Autodesk Inventor part; units mm, degrees
ref_plane "YZ Plane" through (0, 0, 0) normal (1, 0, 0) x (0, 1, 0)
ref_plane "XZ Plane" through (0, 0, 0) normal (0, 1, 0) x (-1, 0, 0)
ref_plane "XY Plane" through (0, 0, 0) normal (0, 0, 1) x (1, 0, 0)
sketch "Sketch1" plane through (0, 0, 0) normal (1, 0, 0) x (0, 1, 0)
  circle A0 centre (0, 0) radius 2.5
  line L0 (2.3039, 4.0032) -> (4.6188, 0.0063)
  line L1 (4.6188, 0.0063) -> (2.3149, -3.9968)
  line L2 (2.3149, -3.9968) -> (-2.3039, -4.0032)
  line L3 (-2.3039, -4.0032) -> (-4.6188, -0.0063)
  line L4 (-4.6188, -0.0063) -> (-2.3149, 3.9968)
  line L5 (-2.3149, 3.9968) -> (2.3039, 4.0032)
  dimension "d0" = 5
  dimension "d1" = 8
extrude "Extrusion1" add sketch "Sketch1" along normal blind 30 contours A0
extrude "Extrusion2" add sketch "Sketch1" against normal blind 5 contours A0 | L0 L1 L2 L3 L4 L5
thread "Thread1"
fillet "Fillet1" radius 0.5 6 edges at (-2.5, 2.3039, 4.0032) (-2.5, 4.6188, 0.0063) (-2.5, -2.3149, 3.9968) (-2.5, -4.6188, -0.0063) (-2.5, -2.3039, -4.0032) (-2.5, 2.3149, -3.9968)
fillet "Fillet2" radius 0.5 24 edges at (-5, -4.5414, -0.0062) (-5, -3.4668, 1.9953) (-5, -2.2761, 3.9299) (-5, -0.0055, 4) (-5, 2.2653, 3.9361) (-5, 3.4614, 2.0047) (-5, 4.5414, 0.0062) (-5, 3.4668, -1.9953) (-5, 2.2761, -3.9299) (-5, 0.0055, -4) (-5, -2.2653, -3.9361) (-5, -3.4614, -2.0047) (0, -4.5414, -0.0062) (0, -3.4668, 1.9953) (0, -2.2761, 3.9299) (0, -0.0055, 4) (0, 2.2653, 3.9361) (0, 3.4614, 2.0047) (0, 4.5414, 0.0062) (0, 3.4668, -1.9953) (0, 2.2761, -3.9299) (0, 0.0055, -4) (0, -2.2653, -3.9361) (0, -3.4614, -2.0047)
fillet "Fillet3" radius 0.5 2 edges at (0, -2.5, 0) (30, -2.5, 0)
properties part number "SzenzorCsavar5os"
Could you check a few things on this model? Use its own coordinates, in mm. A direction names the side the tool comes from. Coordinates: 2 decimals unless noted, no trailing zeros. Loops run counter-clockwise (first coordinate to the right, second up) from the corner with the lowest first, then second, coordinate; pieces in that order, holes last. Notation, with made-up numbers: (86, 39.25) -> (98, 39.25) arc R28 cw to (98, 64.25) -> close; hole circle Ø8 at (59, 36.5). An arc over 180 degrees is marked (long way). Answer in a Markdown table with one row per item.
(1) Imagine slicing it at A-A (x = 6). List the corners of the cut face in (y, z) for me.
Results found:
| item | result |
|---|---|
| outline | circle Ø5 at (0, 0) |
(2) For faces 1 (the face through (-0.143, 3.351, -1.896)), 2 (the face through (0, 1, 3)), which set-ups out of +Z, -Z, +X, -X, +Y, -Y let a thin tool reach every point of the face, with its end or its side?
Results found:
| item | result |
|---|---|
| face 1 | -Z, +X, +Y |
| face 2 | +X |
(3) If I drill on probe 1 along Z at (x, y) = (-1.5, -0.75); probe 2 along Y at (x, z) = (23, 0.5); probe 3 along X at (y, z) = (3, -0.25), over which ranges is the centre line in solid material (lowest first)?
Results found:
| item | result |
|---|---|
| probe 1 | z = -4 to 4 |
| probe 2 | y = -2.45 to 2.45 |
| probe 3 | x = -5 to 0 |
(4) Will these pins go through, and if not, where does the flat tip stop? pin 1 Ø2 at (x, z) = (9.5, 0) entering from +Y; pin 2 Ø1.5 at (x, y) = (9.5, -0.5) entering from -Z.
Results found:
| item | result |
|---|---|
| pin 1 | stops at y = 2.5 |
| pin 2 | stops at z = -2.5 |
